from build123d import *

# Parameters (mm, degrees)
F0_R     = 2
F1_DEPTH = 5


with BuildPart() as f1:
    # F0 (on Top) → F1 (new body)
    with BuildSketch(Plane.XY):
        with BuildLine():
            Line((-5, -4), (5, -4))
            Line((5, -4), (5, 0))
            ThreePointArc((5, 0), (3.828427, 2.828427), (1, 4))
            Line((1, 4), (-1, 4))
            ThreePointArc((-1, 4), (-3.828427, 2.828427), (-5, 0))
            Line((-5, 0), (-5, -4))
        make_face()
        Circle(F0_R, mode=Mode.SUBTRACT)
    extrude(amount=F1_DEPTH)


solid = f1.part
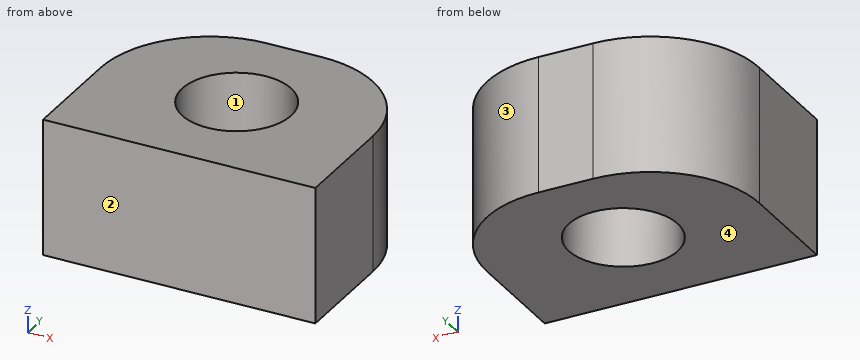
Model file for the job. Use its own axes, mm. Face numbers are marked on the shaded views. Round coordinates to 2 decimals unless told otherwise and drop trailing zeros. Loops run counter-clockwise (first coordinate to the right, second up) from the corner with the lowest first, then second, coordinate; pieces in that order, holes last.
1. Mould opens along Y. For the marked faces 1, 2, 3 and 4 say: +Y half, -Y half, draft (parallel to the pull), parting line (faces both ways), or undercut.
Check values:
face 1: undercut
face 2: -Y half
face 3: +Y half
face 4: draft
2. Band-saw the part on C-C, the plane y = -0.75. List the corners of the cut face in (x, z).
Check values:
outline: (-5, 0) - (-1.85, 0) - (-1.85, 5) - (-5, 5) - close; (1.85, 0) - (5, 0) - (5, 5) - (1.85, 5) - close
3. Band-saw the part on A-A, the plane z = 1.85. List the corners of the cut face in (x, y).
Check values:
outline: (-5, -4) - (5, -4) - (5, 0) arc R4 ccw to (1, 4) - (-1, 4) arc R4 ccw to (-5, 0) - close; hole circle Ø4 at (0, 0)
4. Wall check: probe 1 along Y at (x, z) = (0, 1.45); probe 2 along X at (y, z) = (0.75, 3.45); probe 3 along X at (y, z) = (-1.5, 2.7). Give the ranges that are in metal, low to high.
Check values:
probe 1: y = -4 to -2, 2 to 4
probe 2: x = -4.93 to -1.85, 1.85 to 4.93
probe 3: x = -5 to -1.32, 1.32 to 5
5. Band-saw the part on D-D, the plane x = -3. List the corners of the cut face in (y, z), and give its area (3 significant figures).
Check values:
outline: (-4, 0) - (3.46, 0) - (3.46, 5) - (-4, 5) - close
area: 37.3 mm2
6. Band-saw the part on B-B, the plane x = 0. List the corners of the cut face in (y, z).
Check values:
outline: (-4, 0) - (-2, 0) - (-2, 5) - (-4, 5) - close; (2, 0) - (4, 0) - (4, 5) - (2, 5) - close
